```python
from build123d import *

# Parameters (mm, degrees)
F0_W     = 30
F0_H     = 20
F1_DEPTH = 5
F3_DEPTH = 30
F5_DEPTH = 25.4
F6_W     = 5.25
F6_H     = 17.6155281281
F7_DEPTH = 8
F8_R     = 5.08


with BuildPart() as f1:
    # F0 (on Top) → F1 (new body)
    with BuildSketch(Plane.XY):
        with Locations((15, -10)):
            Rectangle(F0_W, F0_H)
    extrude(amount=F1_DEPTH)

    # F2 (on face) → F3 (cut, through all)
    with BuildSketch(Plane.YZ.offset(30)):
        Polygon((-20, 5), (-20, 0), (0, 5), align=None)
    extrude(amount=-F3_DEPTH, mode=Mode.SUBTRACT)

    # F4 (on face) → F5 (cut)
    with BuildSketch(Plane(origin=(0, -1.1764705882, 4.7058823529), x_dir=(1, 0, 0), z_dir=(0, -0.242535625, 0.9701425001))):
        with BuildLine():
            Line((22.9984683846, -19.4028500029), (22.9984683846, -11.9438578146))
            Line((22.9984683846, -11.9438578146), (22.9984683846, -11.6307859351))
            ThreePointArc((22.9984683846, -11.6307859351), (15, -3.7873218748), (7.0015316154, -11.6307859351))
            Line((7.0015316154, -11.6307859351), (6.8494265755, -19.4028500029))
            Line((6.8494265755, -19.4028500029), (22.9984683846, -19.4028500029))
        make_face()
    extrude(amount=-F5_DEPTH, mode=Mode.SUBTRACT)

    # F6 (on face) → F7 (join)
    with BuildSketch(Plane(origin=(0, -1.1764705882, 4.7058823529), x_dir=(1, 0, 0), z_dir=(0, -0.242535625, 0.9701425001))):
        with Locations((27.375, -10.5950859389)):
            Rectangle(F6_W, F6_H)
        with Locations((2.625, -10.5950859389)):
            Rectangle(F6_W, F6_H)
    extrude(amount=F7_DEPTH)

    # F8
    f8_edges = [f1.edges().sort_by_distance(p)[0] for p in [
        (2.625, -4.850713, 12.033533),
        (27.375, -4.850713, 12.033533),
        (2.625, -21.940285, 7.76114),
        (27.375, -21.940285, 7.76114),
    ]]
    fillet(f8_edges, radius=F8_R)


solid = f1.part
```
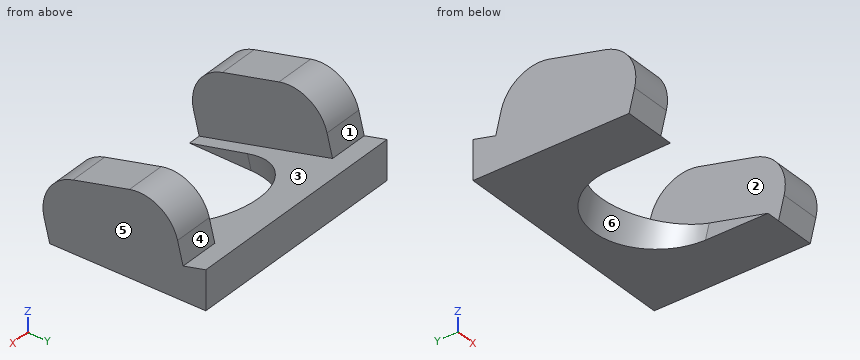
Work out the finished part from the listing and answer in its coordinate system (mm). Face numbers are marked on the shaded views. A direction names the side the tool comes from. Round coordinates to 2 decimals unless told otherwise and drop trailing zeros. Write each loop counter-clockwise with the first axis right and the second up, starting at its lowest first coordinate (ties: lowest second). Pieces come first, ordered by that corner, then holes. Notation, with made-up numbers: (86.25, 80) - (113.25, 80) arc R23 cw to (113.25, 100) - close; hole circle Ø1 at (9.25, 41.25). An arc over 180 degrees is marked (long way). Return JSON: item names as keys, results as strings. Group by question number.
Q1. The part is cut by section A-A on y = -15. Write down the section's boundary in (x, z), then the cut area to 3 significant figures.
Q2. Find the intervals of material crossed by L1, parallel to X at y = -13.5, z = 2.5; L2, parallel to Y at x = 4.75, z = 1.75; L3, parallel to Z at x = 19, y = -4, in increasing order.
Q3. The part is cut by section D-D on y = -3.25. Write down the section's boundary in (x, z).
Q4. For the marked faces 1, 2 and 3, determine the directions among +Z, -Z, +X, -X, +Y, -Y from which every point of the face is accessible in a straight line to the end or side of a thin tool.
Q5. The part is cut by section C-C on x = 2.75. Write down the section's boundary in (y, z).
Q6. This flat-tipped pin is pushed along its axis until it touches: pin 1 Ø10 at (x, y) = (16.5, -8.5) entering from +Z (3 decimals). Where does it stop, or does it pass through?
Q7. The mould has two halves that part along Y. Classify the marked faces 4, 5 and 6: released by +Y, released by -Y, zero draft, split by the parting line, or undercut.
Q8. The part is cut by section B-B on z = 6.5. Write down the section's boundary in (x, y).
Solved:
{
 "1": {"outline": "(0, 0) - (6.94, 0) - (6.95, 1.25) - (5.25, 1.25) - (5.25, 9.5) - (0, 9.5) - close; (23, 0) - (30, 0) - (30, 9.5) - (24.75, 9.5) - (24.75, 1.25) - (23, 1.25) - close", "area": "104 mm²"},
 "2": {"L1": "0 to 5.25, 24.75 to 30", "L2": "-20.44 to 0", "L3": "0 to 4"},
 "3": {"outline": "(0, 0) - (30, 0) - (30, 5.63) - (24.75, 5.63) - (24.75, 4.19) - (5.25, 4.19) - (5.25, 5.63) - (0, 5.63) - close"},
 "4": {"face 1": "+Z, +X, -X", "face 2": "+Z, -Y", "face 3": "+Z"},
 "5": {"outline": "(-20.71, 2.83) - (-20, 0) - (0, 0) - (0, 5) - (-2.91, 4.27) - (-3.62, 7.11) arc R5.08 ccw to (-9.78, 10.8) - (-17.01, 8.99) arc R5.08 ccw to start"},
 "6": {"pin 1": "z = 4.125"},
 "7": {"face 4": "undercut", "face 5": "zero draft", "face 6": "released by -Y"},
 "8": {"outline": "(0, -20.24) - (5.25, -20.24) - (5.25, -3.47) - (0, -3.47) - close; (24.75, -20.24) - (30, -20.24) - (30, -3.47) - (24.75, -3.47) - close"}
}
